Autodesk Inventor part; units mm, degrees
ref_plane "YZ Plane" through (0, 0, 0) normal (1, 0, 0) x (0, 1, 0)
ref_plane "XZ Plane" through (0, 0, 0) normal (0, 1, 0) x (-1, 0, 0)
ref_plane "XY Plane" through (0, 0, 0) normal (0, 0, 1) x (1, 0, 0)
sketch "Base" plane through (0, 0, 0) normal (0, 0, 1) x (1, 0, 0)
  line L0 (-17.0434, 17.78) -> (17.0434, 17.78)
  line L1 (17.0434, 17.78) -> (17.0434, 0)
  line L2 (17.0434, 0) -> (-17.0434, 0)
  line L3 (-17.0434, 0) -> (-17.0434, 17.78)
  circle A0 centre (13.0434, 13.78) radius 4 construction
  circle A1 centre (-13.0434, 13.78) radius 4 construction
  circle A2 centre (-13.0434, 4) radius 4 construction
  circle A3 centre (13.0434, 4) radius 4 construction
  circle A4 centre (-13.0434, 13.78) radius 1.5875
  circle A5 centre (-13.0434, 4) radius 1.5875
  circle A6 centre (13.0434, 13.78) radius 1.5875
  circle A7 centre (13.0434, 4) radius 1.5875
  point P0 (0, 0)
  point P1 (0, 28.2865)
  point P2 (0, 46.7013)
  point P3 (0, 0)
  dimension "d0" = 17.78
  dimension "d1" = 8
  dimension "d2" = 34.0868
  dimension "d3" = 3.175
extrude "Plate1" add sketch "Base" along normal blind 2.54
fillet "BaseROundFeature" radius 1 4 edges at (-17.0434, 17.78, 1.27) (17.0434, 17.78, 1.27) (-17.0434, 0, 1.27) (17.0434, 0, 1.27)
equation "\"d4\" = Thickness"
equation "\"BendRadius\" = Thickness"
equation "\"BendReliefWidth\" = Thickness"
equation "\"BendReliefDepth\" = 0.5 * Thickness"
equation "\"CornerReliefSize\" = 4 * Thickness"
equation "\"MinimumRemnant\" = 2 * Thickness"
equation "\"TransitionRadius\" = BendRadius"
equation "\"JacobiRadiusSize\" = BendRadius"
equation "\"GapSize\" = Thickness"
properties part number "BatteryPlate"
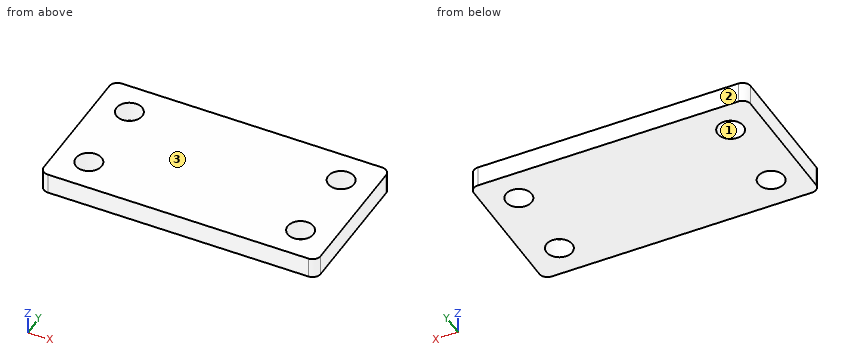
Input: part model. Units: mm. Frame: model coordinates. Face numbers are marked on the shaded views. Coordinates: 2 decimals unless noted, no trailing zeros. Loops run counter-clockwise (first coordinate to the right, second up) from the corner with the lowest first, then second, coordinate; pieces in that order, holes last. Notation, with made-up numbers: (87, 64.25) -> (115, 64.25) arc R26 ccw to (115, 93.25) -> close; hole circle Ø4 at (-36.75, 40). An arc over 180 degrees is marked (long way). Write each question's results on one line, items separated by ' | '. Start each with the question number.
Q1. Pull-direction query (Y, two-part tool) for the marked faces 1, 2 and 3; classes: released by +Y, released by -Y, zero draft, split by the parting line, or undercut.
Q2. Section A-A, the plane y = 13.78. Return the cut outline in (x, z), plus the area to 3 significant figures.
Q3. Section C-C, the plane x = -13. Return the cut outline in (y, z), plus the area to 3 significant figures.
Q4. Section B-B, the plane z = 1.35. Return the cut outline in (x, y) (1 decimal), plus the area to 3 significant figures.
Q5. Ray query, line 1 (Y direction, x = 13, z = 2.4); line 2 (X direction, y = 13, z = 0.95); line 3 (Y direction, x = 12.5, z = 2.35). Return the intervals inside material, ascending. Write a range as from..to.
Found:
1) face 1: undercut | face 2: released by +Y | face 3: zero draft
2) outline: (-17.04, 0) -> (-14.63, 0) -> (-14.63, 2.54) -> (-17.04, 2.54) -> close; (-11.46, 0) -> (11.46, 0) -> (11.46, 2.54) -> (-11.46, 2.54) -> close; (14.63, 0) -> (17.04, 0) -> (17.04, 2.54) -> (14.63, 2.54) -> close | area: 70.5 mm2
3) outline: (0, 0) -> (2.41, 0) -> (2.41, 2.54) -> (0, 2.54) -> close; (5.59, 0) -> (12.19, 0) -> (12.19, 2.54) -> (5.59, 2.54) -> close; (15.37, 0) -> (17.78, 0) -> (17.78, 2.54) -> (15.37, 2.54) -> close | area: 29.0 mm2
4) outline: (-17, 1) arc R1 ccw to (-16, 0) -> (16, 0) arc R1 ccw to (17, 1) -> (17, 16.8) arc R1 ccw to (16, 17.8) -> (-16, 17.8) arc R1 ccw to (-17, 16.8) -> close; hole circle Ø3.2 at (-13, 4); hole circle Ø3.2 at (-13, 13.8); hole circle Ø3.2 at (13, 4); hole circle Ø3.2 at (13, 13.8) | area: 574 mm2
5) line 1: 0..2.41, 5.59..12.19, 15.37..17.78 | line 2: -17.04..-14.43, -11.66..11.66, 14.43..17.04 | line 3: 0..2.51, 5.49..12.29, 15.27..17.78
